The listing builds one solid part. Answer for the finished solid, in the listing's coordinates (mm). A direction names the side the tool comes from. Coordinates: 2 decimals unless noted, no trailing zeros. Loops run counter-clockwise (first coordinate to the right, second up) from the corner with the lowest first, then second, coordinate; pieces in that order, holes last. Notation, with made-up numbers: (65, 23.25) - (95, 23.25) arc R25 ccw to (95, 59.25) - close; hole circle Ø9 at (-18, 8). An arc over 180 degrees is marked (long way). Put each result on its own line as item: value.
Autodesk Inventor part; units mm, degrees
ref_plane "Work Plane1" through (0, 7.749, 0) normal (0, 1, 0) x (-1, 0, 0)
ref_plane "Work Plane2" through (0, 16.1, 0) normal (0, 1, 0) x (-1, 0, 0)
ref_plane "Work Plane3" through (0, 113.3, 0) normal (0, 1, 0) x (-1, 0, 0)
sketch "Sketch1" plane through (0, 0, 0) normal (0, 1, 0) x (-1, 0, 0)
  circle A0 centre (0, 0) radius 27
  circle A1 centre (0, 0) radius 31.877
  dimension "d0" = 54
  dimension "d1" = 63.754
extrude "Extrusion1" add sketch "Sketch1" along normal blind 114.2
ref_plane "Work Plane1" through (0, 7.749, 0) normal (0, 1, 0) x (-1, 0, 0)
sketch "Sketch3" plane through (0, 7.749, 0) normal (0, 1, 0) x (-1, 0, 0)
  circle A0 centre (0, 0) radius 31.877
  circle A1 centre (0, 0) radius 30.988
  dimension "d6" = 61.976
extrude "Extrusion2" cut sketch "Sketch3" along normal blind 200
ref_plane "Work Plane2" through (0, 16.1, 0) normal (0, 1, 0) x (-1, 0, 0)
sketch "Sketch4" plane through (0, 16.1, 0) normal (0, 1, 0) x (-1, 0, 0)
  circle A0 centre (0, 0) radius 28
  circle A1 centre (0, 0) radius 26.4727
  circle A2 centre (0, 0) radius 31.5514
  dimension "d10" = 56
extrude "Extrusion3" cut sketch "Sketch4" along normal blind 200 contours A2
ref_plane "Work Plane3" through (0, 113.3, 0) normal (0, 1, 0) x (-1, 0, 0)
properties part number "Vacuum Cylinder"
1) For faces 4 (the face through (-16.66, 11.87, -26.13)), 5 (the face through (-30.405, 3.82, -9.575)), determine the directions among +Z, -Z, +X, -X, +Y, -Y from which every point of the face is accessible in a straight line to the end or side of a thin tool.
Found:
face 4: +Y
face 5: +Y, -Y
2) The part is cut by section C-C (y = 50). Give the vertices of the cut face in (x, z), and give its area (3 significant figures).
Found:
outline: circle Ø56 at (0, 0); hole circle Ø54 at (0, 0)
area: 173 mm^2
3) Straight lines are drawn through the part: L1, parallel to Z at x = 0, y = 42; L2, parallel to X at y = 36.5, z = 17.5; L3, parallel to X at y = 19.5, z = -14.5. For each, find the intervals that lie inside material, in ascending order. Write a range as [from, to].
Found:
L1: z = [-28, -27], [27, 28]
L2: x = [-21.86, -20.56], [20.56, 21.86]
L3: x = [-23.95, -22.78], [22.78, 23.95]
4) Each of these flat-tipped pins is pushed along its axis until it touches: pin 1 (3 mm diameter, centred on y = 25, z = -22, fed in from +X); pin 2 (12 mm diameter, centred on y = 26, z = -2, fed in from +X); pin 3 (6 mm diameter, centred on x = -22.5, y = 63.5, fed in from +Z). Where does it stop, or does it pass through?
Found:
pin 1: stops at x = 19.07
pin 2: stops at x = 28
pin 3: stops at z = 20.09
5) For a pull along Z with two mould halves and no side action, classify faces 1 (the face through (-25.865, 64.463, 10.724)), 2 (the face through (31, 7.749, 5)), 3 (the face through (5.85, 56.3, 26.36)) as pulls with the +Z half, pulls with the -Z half, needs draft (parallel to the pull), parting line crosses it, or undercut.
Found:
face 1: parting line crosses it
face 2: needs draft
face 3: undercut
6) The part is cut by section A-A (z = 0). Give the vertices of the cut face in (x, y).
Found:
outline: (-31.88, 0) - (-27, 0) - (-27, 114.2) - (-28, 114.2) - (-28, 16.1) - (-30.99, 16.1) - (-30.99, 7.75) - (-31.88, 7.75) - close; (27, 0) - (31.88, 0) - (31.88, 7.75) - (30.99, 7.75) - (30.99, 16.1) - (28, 16.1) - (28, 114.2) - (27, 114.2) - close
7) The part is cut by section B-B (x = 0). Give the vertices of the cut face in (y, z), and give its area (3 significant figures).
Found:
outline: (0, -31.88) - (7.75, -31.88) - (7.75, -30.99) - (16.1, -30.99) - (16.1, -28) - (114.2, -28) - (114.2, -27) - (0, -27) - close; (0, 27) - (114.2, 27) - (114.2, 28) - (16.1, 28) - (16.1, 30.99) - (7.75, 30.99) - (7.75, 31.88) - (0, 31.88) - close
area: 338 mm^2
